Read the model definition and answer for the solid it produces. Units are mm, in the model's axes. A direction names the side the tool comes from. Give positions to 0.01 mm unless a question says otherwise; leave off trailing zeros. Order: outer loops, then holes, each group sorted by start corner. A loop starts at its lowest first (then second) coordinate and runs counter-clockwise, first axis right, second up. Notation, with made-up numbers: (78.5, 21) -> (94.5, 21) arc R12 ccw to (94.5, 42) -> close; hole circle Ø3 at (84, 27). An arc over 180 degrees is marked (long way). Answer as CSV lines item,"result". Start each with the question number.
1) Straight lines are drawn through the part: L1, parallel to Z at x = 30, y = -3.5; L2, parallel to X at y = 1, z = 44; L3, parallel to Z at x = 6, y = -4. For each, find the intervals that lie inside material, in ascending order. Write a range as from..to.
2) Find section D-D (x = -32). Determine the outline of the cut face in (y, z), and give its area (3 significant figures).
3) Find section A-A (y = 0). Determine the outline of the cut face in (x, z), and give its area (3 significant figures).
4) Find section C-C (z = 27). Determine the outline of the cut face in (x, y).
5) Find section B-B (x = 2). Determine the outline of the cut face in (y, z), and give its area (3 significant figures).
6) Flat-ended cylindrical pins translate along their axes: pin 1 Ø1.5 at (x, y) = (35.5, -27) entering from +Z; pin 2 Ø3 at (x, y) = (-12.5, 7) entering from +Z; pin 3 Ø5 at (x, z) = (-11.5, 36.5) entering from -Y. Find the tip coordinate at first contact, or state that the pin passes through.
7) For faces 1 (the face through (-0.266, 0.266, 39.405)), 2 (the face through (-18.994, 0.836, 34.168)), determine the directions among +Z, -Z, +X, -X, +Y, -Y from which every point of the face is accessible in a straight line to the end or side of a thin tool.
```python
from build123d import *

# Parameters (mm, degrees)
F0_W          = 100.2360209823
F0_H          = 75.6767615676
F1_DEPTH      = 25.4
F2_R          = 19.0125799506
F3_DEPTH      = 25.4
F5_DEPTH      = 37.8393807838
F5_DEPTH_BACK = 37.8393807838


with BuildPart() as f1:
    # F0 (on Top) → F1 (new body)
    with BuildSketch(Plane.XY):
        Rectangle(F0_W, F0_H)
    extrude(amount=F1_DEPTH)

    # F2 (on face) → F3 (join)
    with BuildSketch(Plane.XY.offset(25.4)):
        Circle(F2_R)
    extrude(amount=F3_DEPTH)

    # F4 (on Front) → F5 (cut, two sides)
    with BuildSketch(Plane.XZ) as f5_sk:
        Polygon((-21.6138623655, 59.192981571), (-21.6138623655, 49.6012866497), (21.2963428348, 29.1053559631), (21.2963428348, 59.192981571), align=None)
    extrude(amount=-F5_DEPTH, mode=Mode.SUBTRACT)
    extrude(f5_sk.sketch, amount=F5_DEPTH_BACK, mode=Mode.SUBTRACT)


solid = f1.part
```
Findings below:
1,L1,"0..25.4"
1,L2,"-18.99..-9.89"
1,L3,"0..36.41"
2,outline,"(-37.84, 0) -> (37.84, 0) -> (37.84, 25.4) -> (-37.84, 25.4) -> close"
2,area,"1,920 mm²"
3,outline,"(-50.12, 0) -> (50.12, 0) -> (50.12, 25.4) -> (19.01, 25.4) -> (19.01, 30.2) -> (-19.01, 48.36) -> (-19.01, 25.4) -> (-50.12, 25.4) -> close"
3,area,"3,070 mm²"
4,outline,"circle Ø38.03 at (0, 0)"
5,outline,"(-37.84, 0) -> (37.84, 0) -> (37.84, 25.4) -> (18.91, 25.4) -> (18.91, 38.32) -> (-18.91, 38.32) -> (-18.91, 25.4) -> (-37.84, 25.4) -> close"
5,area,"2,410 mm²"
6,pin 1,"z = 25.4"
6,pin 2,"z = 45.96"
6,pin 3,"y = -16.75"
7,face 1,"+Z, +X, +Y, -Y"
7,face 2,"+Z"
